from build123d import *

# Parameters (mm, degrees)
F0_R     = 11.25
F1_DEPTH = 7


with BuildPart() as f1:
    # F0 (on Top) → F1 (new body)
    with BuildSketch(Plane.XY):
        with BuildLine():
            ThreePointArc((2.528072, -13.006589), (10.223978, -8.428094), (13.25, 0))
            ThreePointArc((13.25, 0), (13.068272, 2.186954), (12.528072, 4.313919))
            ThreePointArc((12.528072, 4.313919), (11.474837, 6.625), (10, 8.692669))
            ThreePointArc((10, 8.692669), (0, 13.25), (-10, 8.692669))
            ThreePointArc((-10, 8.692669), (-11.474837, 6.625), (-12.528072, 4.313919))
            ThreePointArc((-12.528072, 4.313919), (-11.474837, -6.625), (-2.528072, -13.006589))
            ThreePointArc((-2.528072, -13.006589), (0, -13.25), (2.528072, -13.006589))
        make_face()
        Circle(F0_R, mode=Mode.SUBTRACT)
        with BuildLine():
            ThreePointArc((12.528072, 4.313919), (13.068272, 2.186954), (13.25, 0))
            ThreePointArc((13.25, 0), (10.223978, -8.428094), (2.528072, -13.006589))
            Line((2.528072, -13.006589), (22.112944, -24.313919))
            ThreePointArc((22.112944, -24.313919), (23.16618, -13.375), (32.112944, -6.993411))
            Line((32.112944, -6.993411), (12.528072, 4.313919))
        make_face()
        with BuildLine():
            ThreePointArc((-10, 8.692669), (0, 13.25), (10, 8.692669))
            Line((10, 8.692669), (10, 31.307331))
            ThreePointArc((10, 31.307331), (0, 26.75), (-10, 31.307331))
            Line((-10, 31.307331), (-10, 8.692669))
        make_face()
        with BuildLine():
            ThreePointArc((47.891016, -20), (43.06911, -9.776022), (32.112944, -6.993411))
            ThreePointArc((32.112944, -6.993411), (23.16618, -13.375), (22.112944, -24.313919))
            ThreePointArc((22.112944, -24.313919), (36.827971, -33.068272), (47.891016, -20))
        make_face()
        with Locations((34.641016, -20)):
            Circle(F0_R, mode=Mode.SUBTRACT)
        with BuildLine():
            Line((-22.112944, -24.313919), (-2.528072, -13.006589))
            ThreePointArc((-2.528072, -13.006589), (-11.474837, -6.625), (-12.528072, 4.313919))
            Line((-12.528072, 4.313919), (-32.112944, -6.993411))
            ThreePointArc((-32.112944, -6.993411), (-24.417038, -11.571906), (-21.391016, -20))
            ThreePointArc((-21.391016, -20), (-21.572744, -22.186954), (-22.112944, -24.313919))
        make_face()
        with BuildLine():
            ThreePointArc((-10, 31.307331), (0, 26.75), (10, 31.307331))
            ThreePointArc((10, 31.307331), (12.410933, 35.359822), (13.25, 40))
            ThreePointArc((13.25, 40), (-4.640178, 52.410933), (-10, 31.307331))
        make_face()
        with Locations((0, 40)):
            Circle(F0_R, mode=Mode.SUBTRACT)
        with BuildLine():
            ThreePointArc((-32.112944, -6.993411), (-46.115853, -26.625), (-22.112944, -24.313919))
            ThreePointArc((-22.112944, -24.313919), (-21.572744, -22.186954), (-21.391016, -20))
            ThreePointArc((-21.391016, -20), (-24.417038, -11.571906), (-32.112944, -6.993411))
        make_face()
        with Locations((-34.641016, -20)):
            Circle(F0_R, mode=Mode.SUBTRACT)
    extrude(amount=F1_DEPTH)


solid = f1.part
Work out the finished part from the listing and answer in its coordinate system (mm). A direction names the side the tool comes from. Give positions to 0.01 mm unless a question says otherwise; leave off trailing zeros. Loops run counter-clockwise (first coordinate to the right, second up) from the corner with the lowest first, then second, coordinate; pieces in that order, holes last. Notation, with made-up numbers: (-14, 22.25) - (25, 22.25) arc R23 ccw to (25, 58.25) - close; hole circle Ø10 at (-19, -5). An arc over 180 degrees is marked (long way). Answer in a Markdown table with one row per item.
(1) Section C-C (x = 0) is taken. Give the vertices of the cut face in (y, z).
Results list:
| item | result |
|---|---|
| outline | (-13.25, 0) - (-11.25, 0) - (-11.25, 7) - (-13.25, 7) - close; (11.25, 0) - (28.75, 0) - (28.75, 7) - (11.25, 7) - close; (51.25, 0) - (53.25, 0) - (53.25, 7) - (51.25, 7) - close |
(2) Flat-ended cylindrical pins translate along their axes: pin 1 Ø6 at (x, y) = (0, -13.5) entering from -Z; pin 2 Ø2 at (y, z) = (-5, 4) entering from -X; pin 3 Ø2 at (y, z) = (14, 5) entering from +X. Find the tip coordinate at first contact, or state that the pin passes through.
Results list:
| item | result |
|---|---|
| pin 1 | stops at z = 0 |
| pin 2 | stops at x = -30.39 |
| pin 3 | stops at x = 10 |
(3) For a pull along X with two mould halves and no side action, classify faces 5 (the face through (11.493, 6.594, 3.451)), 6 (the face through (5.19, -9.98, 3.45)), 7 (the face through (-7, -9, 7)) as pulls with the +X half, pulls with the -X half, needs draft (parallel to the pull), parting line crosses it, or undercut.
Results list:
| item | result |
|---|---|
| face 5 | pulls with the +X half |
| face 6 | undercut |
| face 7 | needs draft |
(4) Section A-A (z = 1.25) is taken. Give the vertices of the cut face in (x, y).
Results list:
| item | result |
|---|---|
| outline | (-32.11, -6.99) arc R13.25 ccw (long way) to (-22.11, -24.31) - (-2.53, -13.01) arc R13.25 ccw to (2.53, -13.01) - (22.11, -24.31) arc R13.25 ccw to (47.89, -20) arc R13.25 ccw to (32.11, -6.99) - (12.53, 4.31) arc R13.25 ccw to (10, 8.69) - (10, 31.31) arc R13.25 ccw to (13.25, 40) arc R13.25 ccw (long way) to (-10, 31.31) - (-10, 8.69) arc R13.25 ccw to (-12.53, 4.31) - close; hole circle Ø22.5 at (-34.64, -20); hole circle Ø22.5 at (0, 0); hole circle Ø22.5 at (0, 40); hole circle Ø22.5 at (34.64, -20) |
(5) Section D-D (x = -29) is taken. Give the vertices of the cut face in (y, z), and give its area (3 significant figures).
Results list:
| item | result |
|---|---|
| outline | (-31.99, 0) - (-29.73, 0) - (-29.73, 7) - (-31.99, 7) - close; (-10.27, 0) - (-5.2, 0) - (-5.2, 7) - (-10.27, 7) - close |
| area | 51.3 mm² |
(6) A tool of negligible diameter and unlimited length cuts with its end or side. For faces 1 (the face through (-10, 20, 3)), 2 (the face through (-12.46, -18.74, 3.45)), 3 (the face through (-7, -9, 0)), 4 (the face through (10, 20, 3)), from which of +Z, -Z, +X, -X, +Y, -Y can it reach the whole face along a straight path? Write none if from no direction.
Results list:
| item | result |
|---|---|
| face 1 | +Z, -Z, -X |
| face 2 | +Z, -Z, -Y |
| face 3 | -Z, +X, -X, +Y, -Y |
| face 4 | +Z, -Z, +X |
(7) Section B-B (y = 0) is taken. Give the vertices of the cut face in (x, z).
Results list:
| item | result |
|---|---|
| outline | (-20, 0) - (-11.25, 0) - (-11.25, 7) - (-20, 7) - close; (11.25, 0) - (20, 0) - (20, 7) - (11.25, 7) - close |
(8) Consider L1, parallel to Y at x = 0, z = 2.5; L2, parallel to Y at x = -7.5, z = 2; L3, parallel to X at y = -16, z = 4. Determine where each line is inside the solid, lowest interval first. Write a range as [from, to].
Results list:
| item | result |
|---|---|
| L1 | y = [-13.25, -11.25], [11.25, 28.75], [51.25, 53.25] |
| L2 | y = [-15.88, -8.39], [8.39, 31.61], [48.39, 50.92] |
| L3 | x = [-47.27, -45.16], [-24.13, -7.71], [7.71, 24.13], [45.16, 47.27] |
